Part model, mm, in its own coordinate system. Face numbers are marked on the shaded views. Coordinates: 2 decimals unless noted, no trailing zeros. Loops run counter-clockwise (first coordinate to the right, second up) from the corner with the lowest first, then second, coordinate; pieces in that order, holes last. Notation, with made-up numbers: (81.25, -14) - (101.25, -14) arc R21 cw to (101.25, 1) - close; hole circle Ø7 at (65, 65.5). An arc over 180 degrees is marked (long way). One line per question, with ' | ' between items. Start each with the question number.
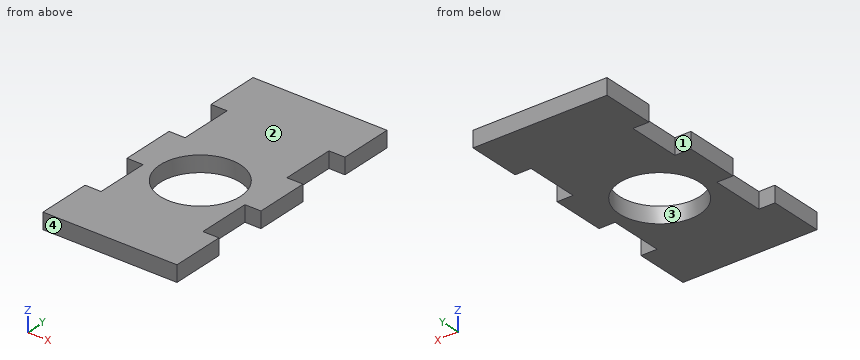
from build123d import *

# Parameters (mm, degrees)
SKETCH1_W           = 25
SKETCH1_H           = 50
BOSS_EXTRUDE1_DEPTH = 3
SKETCH2_R           = 7.5
SKETCH2_W           = 3
SKETCH2_H           = 10
CUT_EXTRUDE1_DEPTH  = 4


with BuildPart() as part:
    # Sketch1 → Boss-Extrude1 (new body)
    with BuildSketch(Plane.XY):
        Rectangle(SKETCH1_W, SKETCH1_H)
    extrude(amount=BOSS_EXTRUDE1_DEPTH)

    # Sketch2 → Cut-Extrude1 (cut, through all)
    with BuildSketch(Plane.XY.offset(3)):
        with Locations((0, -3.5)):
            Circle(SKETCH2_R)
        with Locations((11, 10)):
            Rectangle(SKETCH2_W, SKETCH2_H)
        with Locations((11, -10)):
            Rectangle(SKETCH2_W, SKETCH2_H)
        with Locations((-11, -10)):
            Rectangle(SKETCH2_W, SKETCH2_H)
        with Locations((-11, 10)):
            Rectangle(SKETCH2_W, SKETCH2_H)
    extrude(amount=-CUT_EXTRUDE1_DEPTH, mode=Mode.SUBTRACT)


solid = part.part
1) Pin check, flat tips, straight feed: pin 1 Ø13.5 at (x, y) = (0, -3.5) entering from +Z; pin 2 Ø1.5 at (y, z) = (8, 1.5) entering from +X; pin 3 Ø2 at (x, y) = (-3.5, 17) entering from -Z; pin 4 Ø1.5 at (y, z) = (11, 2) entering from -X. Stop position of each tip, or through.
2) Band-saw the part on B-B on x = 0. List the corners of the cut face in (y, z).
3) Band-saw the part on A-A on y = 1. List the corners of the cut face in (x, z).
4) Mould opens along Y. For the marked faces 1, 2, 3 and 4 say: +Y half, -Y half, draft (parallel to the pull), parting line (faces both ways), or undercut.
5) Wall check: line 1 along Y through (x, z) = (0, 1.25); line 2 along Y through (x, z) = (-6, 2.7); line 3 along X through (y, z) = (-10, 2.2). Give the ranges that are in metal, low to high. Write a range as [from, to].
6) Band-saw the part on D-D on y = 9.5. List the corners of the cut face in (x, z), then the cut area to 3 significant figures.
7) Band-saw the part on C-C on z = 0.45. List the corners of the cut face in (x, y), then the cut area to 3 significant figures.
Values found:
1) pin 1: through | pin 2: x = 9.5 | pin 3: z = 0 | pin 4: x = -9.5
2) outline: (-25, 0) - (-11, 0) - (-11, 3) - (-25, 3) - close; (4, 0) - (25, 0) - (25, 3) - (4, 3) - close
3) outline: (-12.5, 0) - (-6, 0) - (-6, 3) - (-12.5, 3) - close; (6, 0) - (12.5, 0) - (12.5, 3) - (6, 3) - close
4) face 1: undercut | face 2: draft | face 3: undercut | face 4: -Y half
5) line 1: [-25, -11], [4, 25] | line 2: [-25, -8], [1, 25] | line 3: [-9.5, -3.74], [3.74, 9.5]
6) outline: (-9.5, 0) - (9.5, 0) - (9.5, 3) - (-9.5, 3) - close | area: 57.0 mm²
7) outline: (-12.5, -25) - (12.5, -25) - (12.5, -15) - (9.5, -15) - (9.5, -5) - (12.5, -5) - (12.5, 5) - (9.5, 5) - (9.5, 15) - (12.5, 15) - (12.5, 25) - (-12.5, 25) - (-12.5, 15) - (-9.5, 15) - (-9.5, 5) - (-12.5, 5) - (-12.5, -5) - (-9.5, -5) - (-9.5, -15) - (-12.5, -15) - close; hole circle Ø15 at (0, -3.5) | area: 953 mm²
